from build123d import *

# Parameters (mm, degrees)
BOSS_EXTRUDE1_DEPTH = 3.18
SKETCH4_R           = 3.25
TOP_CUT_DEPTH       = 10
SKETCH7_R           = 1
TOP_CUT_2_DEPTH     = 87.044973388
SKETCH10_R          = 1
TOP_CUT_3_DEPTH     = 10
EXTRUDE_M_DEPTH     = 3.18
CIRCLE_M_COUNT      = 5


with BuildPart() as part:
    # Sketch1 → Boss-Extrude1 (new body)
    with BuildSketch(Plane(origin=(0, 0, 0), x_dir=(1, 0, 0), z_dir=(0, 1, 0))):
        Polygon((-59.925822748, 15.118064705), (-32.896231583, -52.321105303), (39.594833528, -47.454286112), (57.367184482, 22.992743574), (-4.139963679, 61.664583135), align=None)
    extrude(amount=BOSS_EXTRUDE1_DEPTH)

    # Sketch4 → Top Cut (cut)
    with BuildSketch(Plane(origin=(0, 3.18, 0), x_dir=(1, 0, 0), z_dir=(0, 1, 0))):
        with Locations(Location((-21.823160529, -34.709503951, 0), (0, 0, 270))):
            Circle(SKETCH4_R)
        with Locations(Location((23.704051479, -14.903621825, 0), (0, 0, 270))):
            Circle(SKETCH4_R)
        Polygon((-34.496448207, -17.291473653), (0.633517523, 38.582361975), (34.496448207, 17.291473653), (-0.633517523, -38.582361975), align=None)
    extrude(amount=-TOP_CUT_DEPTH, mode=Mode.SUBTRACT)

    # Sketch7 → Top Cut 2 (cut, through all)
    with BuildSketch(Plane(origin=(0, 3.18, 0), x_dir=(1, 0, 0), z_dir=(0, 1, 0))):
        with Locations(Location((-29.026773559, 6.437889154, 0), (0, 0, 270))):
            Circle(SKETCH7_R)
        with Locations(Location((-31.155862391, 3.051596086, 0), (0, 0, 270))):
            Circle(SKETCH7_R)
    extrude(amount=-TOP_CUT_2_DEPTH, mode=Mode.SUBTRACT)

    # Sketch10 → Top Cut 3 (cut)
    with BuildSketch(Plane(origin=(0, 3.18, 0), x_dir=(1, 0, 0), z_dir=(0, 1, 0))):
        with Locations(Location((14.832603244, 36.742262873, 0), (0, 0, 270))):
            Circle(SKETCH10_R)
        with Locations(Location((26.684628983, 29.29045196, 0), (0, 0, 270))):
            Circle(SKETCH10_R)
    extrude(amount=-TOP_CUT_3_DEPTH, mode=Mode.SUBTRACT)

    # Sketch3 → Extrude M (add)
    with BuildSketch(Plane(origin=(0, 3.18, 0), x_dir=(1, 0, 0), z_dir=(0, 1, 0))):
        Polygon((-49.511175703, 27.949382471), (-45.436591686, 23.066006068), (-37.589405077, 29.613529441), (-41.663989094, 34.496905844), align=None)
        Polygon((-26.476381351, 47.169118399), (-22.401797334, 42.285741997), (-14.554610725, 48.83326537), (-18.629194741, 53.716641772), align=None)
    extrude_m = extrude(amount=-EXTRUDE_M_DEPTH)

    # Circle M: Extrude M ×5 about axis
    circle_m_axis = Axis((0, 0, 0), (0, 1, 0))
    for i in range(1, CIRCLE_M_COUNT):
        add(extrude_m.rotate(circle_m_axis, i * 360 / CIRCLE_M_COUNT))


solid = part.part
Read the model definition and answer for the solid it produces. Units are mm, in the model's axes. A direction names the side the tool comes from. Coordinates: 2 decimals unless noted, no trailing zeros. Order: outer loops, then holes, each group sorted by start corner. A loop starts at its lowest first (then second) coordinate and runs counter-clockwise, first axis right, second up. Notation, with made-up numbers: M 32,-18.75 L 72,-18.75 A35 cw 72,15.25 Z; hole C -39.75,70.5 d6. An arc over 180 degrees is marked long. Put each result on its own line as item: value. Start each with the question number.
Item 1: Section A-A, the plane x = -8.5 is taken. Determine the outline of the cut face in (y, z), plus the area to 3 significant figures.
Item 2: Section C-C, the plane y = 1.2 is taken. Count the separate pieces of the cut face and the enclosed holes in it, plus the area to 3 significant figures.
Item 3: For faces 4 (the face through (-51.587, 1.612, 10.021)), 5 (the face through (19.075, 1.612, -48.92)), 6 (the face through (35.844, 1.612, -38.429)), 7 (the face through (-55.3, 1.6, 0.5)), determine the directions among +Z, -Z, +X, -X, +Y, -Y from which every point of the face is accessible in a straight line to the end or side of a thin tool.
Item 4: Given pin 1 Ø1 at (y, z) = (0.5, -44) entering from -X, flat-ended and moving along its own axis, determine where the tip first touches the part or whether it passes through.
Item 5: Consider probe 1 along Z at (x, y) = (24, 2.8); probe 2 along Z at (x, y) = (26, 2.15); probe 3 along X at (y, z) = (3, -36). Determine where each line is inside the solid, lowest interval first. Write a range as [from, to].
Item 6: Section D-D, the plane z = 45 is taken. Determine the outline of the cut face in (x, y).
Item 7: The mould has two halves that part along Z. Classify faces 1 (the face through (-10.28, 1.57, -56.54)), 2 (the face through (-43.81, 1.61, 33.64)), 3 (the face through (48.447, 1.568, 12.365)): +Z half, -Z half, draft (parallel to the pull), parting line (faces both ways), or undercut.
Item 8: Section B-B, the plane x = 6 is taken. Determine the outline of the cut face in (y, z).
Computed:
1. outline: M 0,-58.03 L 3.18,-58.03 L 3.18,-24.06 L 0,-24.06 Z; M 0,33.64 L 3.18,33.64 L 3.18,53.87 L 0,53.87 Z
1. area: 172 mm2
2. separate pieces: 1
2. enclosed holes: 7
2. area: 6,690 mm2
3. face 4: +Z, +Y, -Y
3. face 5: +X, +Y, -Y
3. face 6: -Z, +Y, -Y
3. face 7: -X, +Y, -Y
4. pin 1: stops at x = -25.91
5. probe 1: z = [-43.97, -23.89], [-0.6, 11.67], [18.14, 48.5]
5. probe 2: z = [-42.71, -30.02], [-28.56, -22.63], [-3.78, 12.6], [17.2, 48.37]
5. probe 3: x = [-34.9, -0.99], [4.74, 14.16], [15.5, 42.65]
6. outline: M -35.83,0 L 40.21,0 L 40.21,3.18 L -35.83,3.18 Z
7. face 1: -Z half
7. face 2: +Z half
7. face 3: undercut
8. outline: M 0,-55.29 L 3.18,-55.29 L 3.18,-35.21 L 0,-35.21 Z; M 0,28.03 L 3.18,28.03 L 3.18,49.71 L 0,49.71 Z
